```python
from build123d import *

# Parameters (mm, degrees)
SKETCH1_W           = 200
SKETCH1_H           = 140
BOSS_EXTRUDE1_DEPTH = 3
SKETCH2_R           = 1.5
SKETCH2_R_2         = 2.5
SKETCH2_W           = 70
SKETCH2_H           = 10
CUT_EXTRUDE1_DEPTH  = 3
FILLET1_R           = 10
FILLET2_R           = 20


with BuildPart() as part:
    # Sketch1 → Boss-Extrude1 (new body)
    with BuildSketch(Plane.XY):
        Rectangle(SKETCH1_W, SKETCH1_H)
    extrude(amount=BOSS_EXTRUDE1_DEPTH)

    # Sketch2 → Cut-Extrude1 (cut)
    with BuildSketch(Plane.XY.offset(3)):
        with Locations((3.621068531, -17.5)):
            Circle(SKETCH2_R)
        with Locations((41.621068531, 14)):
            Circle(SKETCH2_R)
        with Locations((-44.111928007, 18.5)):
            Circle(SKETCH2_R)
        with Locations((-7.111928007, 18.5)):
            Circle(SKETCH2_R)
        with Locations((-7.111928007, -18.5)):
            Circle(SKETCH2_R)
        with Locations((61.917005655, -23.5)):
            Circle(SKETCH2_R_2)
        with Locations((92.917005655, -23.5)):
            Circle(SKETCH2_R_2)
        with Locations((92.917005655, 23.5)):
            Circle(SKETCH2_R_2)
        with Locations((61.917005655, 23.5)):
            Circle(SKETCH2_R_2)
        with Locations((-60, 55)):
            Circle(SKETCH2_R_2)
        with Locations((-60, -55)):
            Circle(SKETCH2_R_2)
        with Locations((-80, -55)):
            Circle(SKETCH2_R_2)
        with BuildLine():
            ThreePointArc((46.5, 45), (45, 46.5), (43.5, 45))
            Line((43.5, 45), (45, 45))
            Line((45, 45), (45, 43.5))
            ThreePointArc((45, 43.5), (46.060660172, 43.939339828), (46.5, 45))
        make_face()
        with BuildLine():
            Line((45, 45), (43.5, 45))
            ThreePointArc((43.5, 45), (43.939339828, 43.939339828), (45, 43.5))
            Line((45, 43.5), (45, 45))
        make_face()
        with Locations((-5, 35)):
            Rectangle(SKETCH2_W, SKETCH2_H)
        with BuildLine():
            Line((-45, 43.5), (-45, 45))
            Line((-45, 45), (-43.5, 45))
            ThreePointArc((-43.5, 45), (-46.060660172, 46.060660172), (-45, 43.5))
        make_face()
        with BuildLine():
            Line((-43.5, 45), (-45, 45))
            Line((-45, 45), (-45, 43.5))
            ThreePointArc((-45, 43.5), (-43.939339828, 43.939339828), (-43.5, 45))
        make_face()
        with BuildLine():
            ThreePointArc((-42.611928007, -18.5), (-43.43447247, -17.161697346), (-45, -17.291145941))
            Line((-45, -17.291145941), (-45, -19.708854059))
            ThreePointArc((-45, -19.708854059), (-43.43447247, -19.838302654), (-42.611928007, -18.5))
        make_face()
        with BuildLine():
            Line((-45, -19.708854059), (-45, -17.291145941))
            ThreePointArc((-45, -17.291145941), (-45.611928007, -18.5), (-45, -19.708854059))
        make_face()
        with Locations((41.621068531, -14)):
            Circle(SKETCH2_R)
        with Locations((-80, 55)):
            Circle(SKETCH2_R_2)
        with Locations((-5, -35)):
            Rectangle(SKETCH2_W, SKETCH2_H)
        with Locations((45, -45)):
            Circle(SKETCH2_R)
        with Locations((-45, -45)):
            Circle(SKETCH2_R)
        with Locations((3.621068531, 17.5)):
            Circle(SKETCH2_R)
    extrude(amount=-CUT_EXTRUDE1_DEPTH, mode=Mode.SUBTRACT)

    # Fillet1
    fillet1_edges = [part.edges().sort_by_distance(p)[0] for p in [
        (-100, -70, 1.5),
        (-100, 70, 1.5),
    ]]
    fillet(fillet1_edges, radius=FILLET1_R)

    # Fillet2
    fillet2_edges = [part.edges().sort_by_distance(p)[0] for p in [
        (100, -70, 1.5),
        (100, 70, 1.5),
    ]]
    fillet(fillet2_edges, radius=FILLET2_R)


solid = part.part
```
Check sheet for the modelled part. Datum: model origin and axes. Units: mm. Give positions to 0.01 mm unless a question says otherwise; leave off trailing zeros. Write each loop counter-clockwise with the first axis right and the second up, starting at its lowest first coordinate (ties: lowest second). Pieces come first, ordered by that corner, then holes.
Item 1: Cross-section at A-A (x = 18). Enter the section's corners in (y, z), and give its area (3 significant figures).
Item 2: Cross-section at C-C (z = 0.8). Count the separate pieces of the cut face and the enclosed holes in it, and give its area (3 significant figures).
Item 3: Gauge pin test, flat end, axial feed: pin 1 (5 mm diameter, centred on x = -7.11, y = 18.5, fed in from -Z). Record the tip position at first contact, or that the pin passes through.
Item 4: Draft check along Y on faces 1 (the face through (-1, 1, 0)), 2 (the face through (-97.15, 66.99, 1.52)), 3 (the face through (95.3, 24.25, 1.52)). Enter one of: released by +Y, released by -Y, zero draft, split by the parting line, or undercut.
Item 5: Cross-section at B-B (y = 55). Enter the section's corners in (x, z), and give its area (3 significant figures).
Item 6: Scan lines: L1, parallel to Y at x = -80, z = 1.15; L2, parallel to Y at x = -26, z = 1.7; L3, parallel to Y at x = -45, z = 0.65. Record each from-to range of solid material in increasing order.
Report:
1. outline: (-70, 0) - (-40, 0) - (-40, 3) - (-70, 3) - close; (-30, 0) - (30, 0) - (30, 3) - (-30, 3) - close; (40, 0) - (70, 0) - (70, 3) - (40, 3) - close
1. area: 360 mm2
2. separate pieces: 1
2. enclosed holes: 22
2. area: 26,100 mm2
3. pin 1: stops at z = 0
4. face 1: zero draft
4. face 2: released by +Y
4. face 3: undercut
5. outline: (-100, 0) - (-82.5, 0) - (-82.5, 3) - (-100, 3) - close; (-77.5, 0) - (-62.5, 0) - (-62.5, 3) - (-77.5, 3) - close; (-57.5, 0) - (99.36, 0) - (99.36, 3) - (-57.5, 3) - close
5. area: 568 mm2
6. L1: y = -70 to -57.5, -52.5 to 52.5, 57.5 to 70
6. L2: y = -70 to -40, -30 to 30, 40 to 70
6. L3: y = -70 to -46.5, -43.5 to -19.71, -17.29 to 17.29, 19.71 to 43.5, 46.5 to 70
